from build123d import *

# Parameters (mm, degrees)
SKETCH1_W           = 60
SKETCH1_H           = 10
BOSS_EXTRUDE1_DEPTH = 3


with BuildPart() as part:
    # Sketch1 → Boss-Extrude1 (new body)
    with BuildSketch(Plane.XY):
        with BuildLine():
            Line((0, 0), (120, 0))
            Line((120, 0), (120, 80))
            Line((120, 80), (0, 80))
            ThreePointArc((0, 80), (-40, 40), (0, 0))
        make_face()
        with Locations((85, 70)):
            Rectangle(SKETCH1_W, SKETCH1_H, mode=Mode.SUBTRACT)
        with Locations((85, 10)):
            Rectangle(SKETCH1_W, SKETCH1_H, mode=Mode.SUBTRACT)
        with BuildLine():
            Line((2.5, 55), (2.5, 74.910600109))
            ThreePointArc((2.5, 74.910600109), (35, 40), (2.5, 5.089399891))
            Line((2.5, 5.089399891), (2.5, 25))
            Line((2.5, 25), (-2.5, 25))
            Line((-2.5, 25), (-2.5, 5.089399891))
            ThreePointArc((-2.5, 5.089399891), (-35, 40), (-2.5, 74.910600109))
            Line((-2.5, 74.910600109), (-2.5, 55))
            Line((-2.5, 55), (2.5, 55))
        make_face(mode=Mode.SUBTRACT)
    extrude(amount=BOSS_EXTRUDE1_DEPTH)


solid = part.part
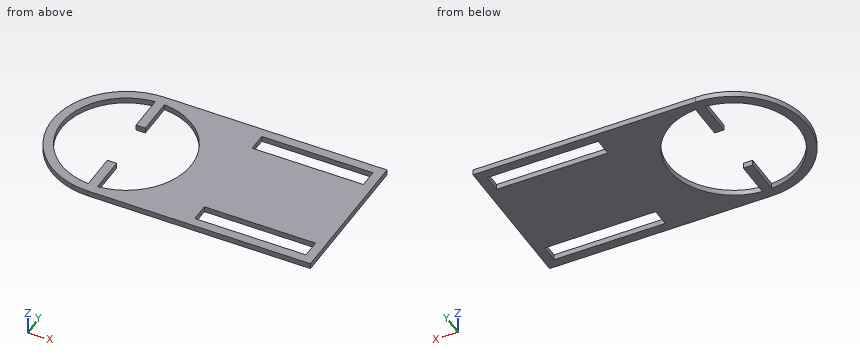
Source: CAD feature listing. Evaluate the final solid. Frame: model axes, mm. Round coordinates to 2 decimals unless told otherwise and drop trailing zeros. Loops run counter-clockwise (first coordinate to the right, second up) from the corner with the lowest first, then second, coordinate; pieces in that order, holes last. Notation, with made-up numbers: (73.5, 4.5) - (122.5, 4.5) arc R18 ccw to (122.5, 25.5) - close; hole circle Ø8 at (55, 79). An arc over 180 degrees is marked (long way). Write item = value, one per line. Start each with the question number.
Item 1: Material intervals for line 1 (Y direction, x = 81.5, z = 2.45); line 2 (X direction, y = 66, z = 2.85); line 3 (X direction, y = 62, z = 2.6), sorted ascending.
Item 2: Section query D-D on y = 61. Output: boundary loops of the cut face in (x, z).
Item 3: Section query C-C on x = 18.5. Output: boundary loops of the cut face in (y, z), plus the area to 3 significant figures.
Item 4: Section query B-B on z = 1.45. Output: boundary loops of the cut face in (x, y), plus the area to 3 significant figures.
Item 5: Section query A-A on y = 40. Output: boundary loops of the cut face in (x, z).
Item 6: First-contact query: pin 1 Ø0.9 at (y, z) = (67.5, 1) entering from -X; pin 2 Ø1.5 at (y, z) = (9, 1.5) entering from -X. Flat tips, straight axial feed; report the tip coordinate or a pass-through.
Results list:
q1.line_1 = 0 to 5, 15 to 65, 75 to 80
q1.line_2 = -30.4 to -23.43, -2.5 to 2.5, 23.43 to 55, 115 to 120
q1.line_3 = -33.41 to -27.22, -2.5 to 2.5, 27.22 to 120
q2.outline = (-34.04, 0) - (-28, 0) - (-28, 3) - (-34.04, 3) - close; (-2.5, 0) - (2.5, 0) - (2.5, 3) - (-2.5, 3) - close; (28, 0) - (120, 0) - (120, 3) - (28, 3) - close
q3.outline = (0, 0) - (10.29, 0) - (10.29, 3) - (0, 3) - close; (69.71, 0) - (80, 0) - (80, 3) - (69.71, 3) - close
q3.area = 61.7 mm²
q4.outline = (0, 0) - (120, 0) - (120, 80) - (0, 80) arc R40 ccw to start; hole (-2.5, 5.09) - (-2.5, 25) - (2.5, 25) - (2.5, 5.09) arc R35 ccw to (2.5, 74.91) - (2.5, 55) - (-2.5, 55) - (-2.5, 74.91) arc R35 ccw to start; hole (55, 5) - (115, 5) - (115, 15) - (55, 15) - close; hole (55, 65) - (115, 65) - (115, 75) - (55, 75) - close
q4.area = 7,260 mm²
q5.outline = (-40, 0) - (-35, 0) - (-35, 3) - (-40, 3) - close; (35, 0) - (120, 0) - (120, 3) - (35, 3) - close
q6.pin_1 = -29.47
q6.pin_2 = -26.17
